Could you check a few things on this drawing? It's one solid part, dimensions in mm from its lowest x, y, z. A direction names the side the tool comes from. Round coordinates to 2 decimals unless told otherwise and drop trailing zeros. Loops run counter-clockwise (first coordinate to the right, second up) from the corner with the lowest first, then second, coordinate; pieces in that order, holes last. Notation, with made-up numbers: (36.5, 51.25) -> (81.5, 51.25) arc R21 ccw to (81.5, 85.25) -> close; hole circle Ø9 at (-7.75, 24.5). An arc over 180 degrees is marked (long way). Write each question's results on one line, items separated by ' | '.
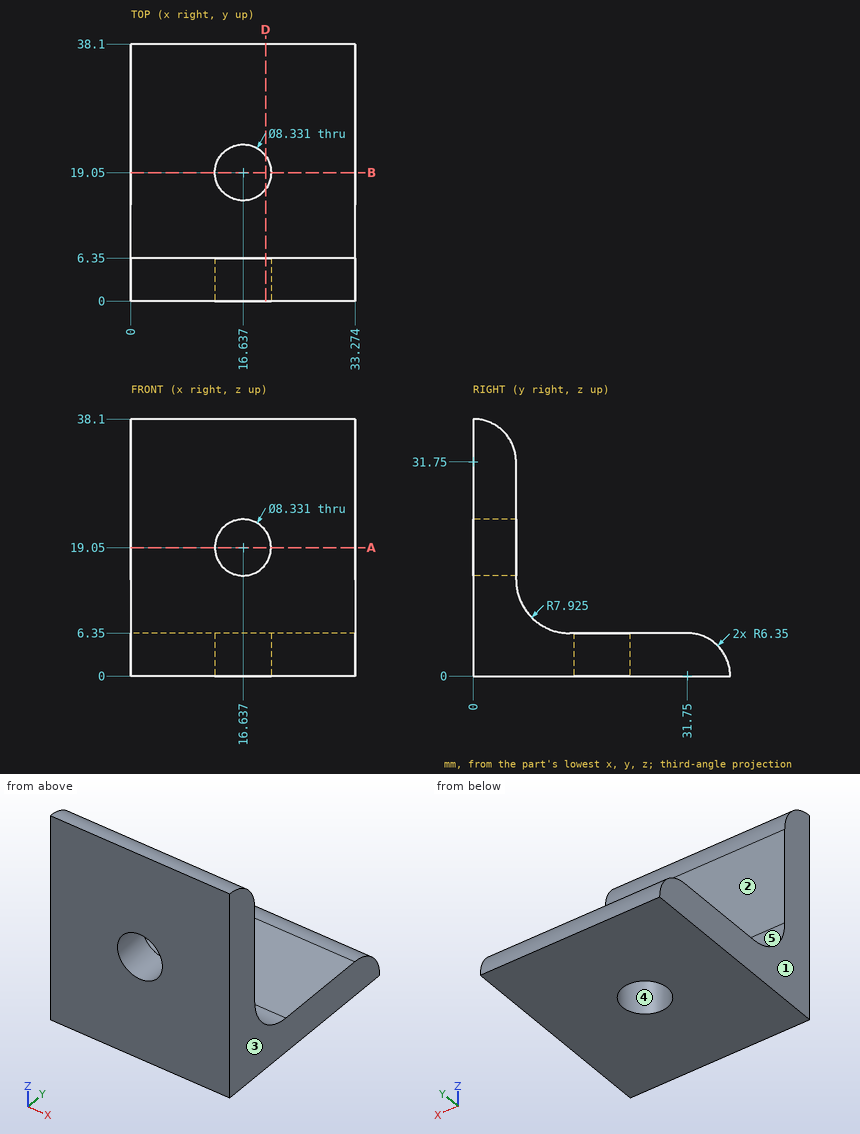
1) I want a section at D-D, the plane x = 20. Give the number of separate pieces and of enclosed holes in the cut face, plus the area to 3 significant figures.
Model answer:
separate pieces: 3 | enclosed holes: 0 | area: 377 mm2
2) I'm going to push flat-ended pins straight in: pin 1 (1.5 mm diameter, centred on x = 27.5, z = 14.5, fed in from +Y); pin 2 (3 mm diameter, centred on x = 20, z = 25.5, fed in from +Y); pin 3 (2 mm diameter, centred on x = 17.5, z = 6.5, fed in from +Y). Where does each tip first touch, or does it pass through?
Model answer:
pin 1: stops at y = 6.37 | pin 2: stops at y = 6.35 | pin 3: stops at y = 34.92
3) I need wall thicknesses on line 1 (X direction, y = 19, z = 4); line 2 (Z direction, x = 9, y = 29). Which ranges of each line are inside material? Lowest first, please.
Model answer:
line 1: x = 0 to 12.47, 20.8 to 33.27 | line 2: z = 0 to 6.35
4) I want a section at A-A, the plane z = 19.05. Write out the boundary of the cut face in (x, y).
Model answer:
outline: (0, 0) -> (12.47, 0) -> (12.47, 6.35) -> (0, 6.35) -> close; (20.8, 0) -> (33.27, 0) -> (33.27, 6.35) -> (20.8, 6.35) -> close
5) For the marked faces 1 and 2, which set-ups out of +Z, -Z, +X, -X, +Y, -Y let a thin tool reach every point of the face, with its end or its side?
Model answer:
face 1: +Z, -Z, -X, +Y, -Y | face 2: +Z, +X, -X, +Y
6) If we mould it in two halves opening along X, with no side actions, what happens to the marked faces 3, 4 and 5? For each: released by +X, released by -X, zero draft, split by the parting line, or undercut.
Model answer:
face 3: released by +X | face 4: undercut | face 5: zero draft
